For this review, take the finished solid that the model builds, in its own axes (mm). Face numbers are marked on the shaded views. A direction names the side the tool comes from. Give positions to 0.01 mm unless a question says otherwise; leave off trailing zeros. Write each loop counter-clockwise with the first axis right and the second up, starting at its lowest first coordinate (ties: lowest second). Pieces come first, ordered by that corner, then holes.
Q1. We need section B-B (y = 14.75). Write out the cut boundary in (x, z).
Q2. For line 1 (Z direction, x = -8, y = 8); line 2 (X direction, y = 3.5, z = -20); line 3 (Z direction, x = -9.5, y = 15.5), list the stretches that pass through material, from the lowest coordinate up.
Q3. Machinability: for the marked faces 5, 6 and 7, which of the approach directions +Z, -Z, +X, -X, +Y, -Y give a long, thin tool a straight path to every point of the face, cutting with its end or side? Answer none if there is none.
Q4. Insertion check: P1, Ø8, axis at x = -8.5, y = 17, coming from the -Z side; P2, Ø12, axis at x = -15.5, y = 9, coming from the -Z side; P3, Ø6, axis at x = -10, z = -13, coming from the +Y side. Each pin has a flat end and moves straight along its axis. Give the tip position at first contact, or say it passes through.
Q5. We need section A-A (x = -8). Write out the cut boundary in (y, z), then the cut area to 3 significant figures.
Q6. We need section D-D (z = -11.5). Write out the cut boundary in (x, y), then the cut area to 3 significant figures.
Q7. Mouldability with a two-part tool opening along Z and no side actions: class the marked faces 1, 2, 3 and 4 as released by +Z, released by -Z, zero draft, split by the parting line, or undercut.
Q8. We need section C-C (y = 8.25). Write out the cut boundary in (x, z).
```python
from build123d import *

# Parameters (mm, degrees)
SKETCH3_R                = 2.5
BOSS_EXTRUDE2_DEPTH      = 10
SKETCH4_W                = 24
SKETCH4_H                = 95
SKETCH4_W_2              = 20
SKETCH4_H_2              = 40.5
BOSS_EXTRUDE3_DEPTH      = 10
BOSS_EXTRUDE3_DEPTH_BACK = 10


with BuildPart() as part:
    # Sketch3 → Boss-Extrude2 (new body)
    with BuildSketch(Plane(origin=(0, 0, 0), x_dir=(1, 0, 0), z_dir=(0, 1, 0))):
        with BuildLine():
            Line((-20, 20), (-20, 7))
            Line((-20, 7), (4, 7))
            Line((4, 7), (4, 20))
            ThreePointArc((4, 20), (-8, 32), (-20, 20))
        make_face()
        with Locations((-8, 20)):
            Circle(SKETCH3_R, mode=Mode.SUBTRACT)
    extrude(amount=BOSS_EXTRUDE2_DEPTH)

    # Sketch4 → Boss-Extrude3 (add, two sides)
    with BuildSketch(Plane(origin=(0, 10, 0), x_dir=(1, 0, 0), z_dir=(0, 1, 0))) as boss_extrude3_sk:
        with Locations((-8, -40.5)):
            Rectangle(SKETCH4_W, SKETCH4_H)
        with Locations((-8, -57.75)):
            Rectangle(SKETCH4_W_2, SKETCH4_H_2, mode=Mode.SUBTRACT)
    extrude(amount=BOSS_EXTRUDE3_DEPTH)
    extrude(boss_extrude3_sk.sketch, amount=-BOSS_EXTRUDE3_DEPTH_BACK)


solid = part.part
```
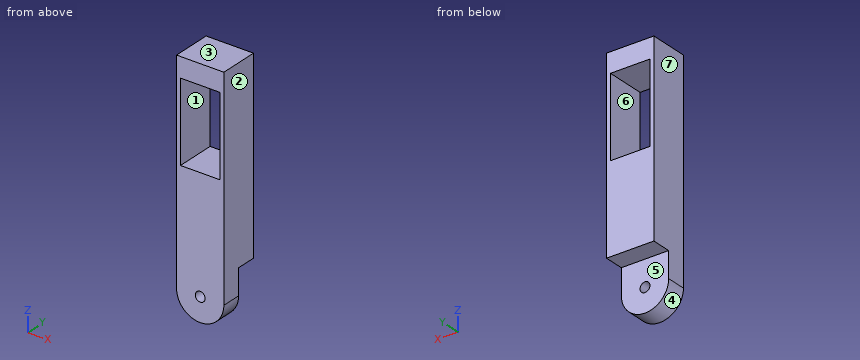
Computed:
1. outline: (-20, -7) - (4, -7) - (4, 88) - (-20, 88) - close; hole (-18, 37.5) - (2, 37.5) - (2, 78) - (-18, 78) - close
2. line 1: z = -32 to -22.5, -17.5 to 37.5, 78 to 88
2. line 2: x = -20 to -10.5, -5.5 to 4
2. line 3: z = -7 to 37.5, 78 to 88
3. face 5: -Z, +X, -X, +Y
3. face 6: +Y, -Y
3. face 7: +Z, -Z, -X, +Y, -Y
4. P1: stops at z = -7
4. P2: stops at z = -31.91
4. P3: stops at y = 10
5. outline: (0, -32) - (10, -32) - (10, -22.5) - (0, -22.5) - close; (0, -17.5) - (10, -17.5) - (10, -7) - (20, -7) - (20, 37.5) - (0, 37.5) - close; (0, 78) - (20, 78) - (20, 88) - (0, 88) - close
5. area: 1,290 mm2
6. outline: (-20, 0) - (4, 0) - (4, 10) - (-20, 10) - close
6. area: 240 mm2
7. face 1: undercut
7. face 2: zero draft
7. face 3: released by +Z
7. face 4: released by -Z
8. outline: (-20, -20) arc R12 ccw to (4, -20) - (4, 88) - (-20, 88) - close; hole (-18, 37.5) - (2, 37.5) - (2, 78) - (-18, 78) - close; hole circle Ø5 at (-8, -20)
